```python
from build123d import *

# Parameters (mm, degrees)
F0_R     = 4.075
F1_DEPTH = 5
F2_R     = 8
F3_R     = 30
F4_W     = 8
F4_H     = 8
F5_DEPTH = 4
F6_R     = 1
F8_COUNT = 3
F8_ANGLE = 180
F9_SIZE  = 0.25


with BuildPart() as f1:
    # F0 (on Top) → F1 (new body)
    with BuildSketch(Plane.XY):
        Polygon((-14.5, 14.5), (-68, 14.5), (-68, -14.5), (0, -14.5), (68, -14.5), (68, 14.5), (14.5, 14.5), (14.5, 68), (-14.5, 68), align=None)
        with Locations((-60, 0)):
            Circle(F0_R, mode=Mode.SUBTRACT)
        with Locations((-30, 0)):
            Circle(F0_R, mode=Mode.SUBTRACT)
        Circle(F0_R, mode=Mode.SUBTRACT)
        with Locations((30, 0)):
            Circle(F0_R, mode=Mode.SUBTRACT)
        with Locations((60, 0)):
            Circle(F0_R, mode=Mode.SUBTRACT)
        with Locations((0, 30)):
            Circle(F0_R, mode=Mode.SUBTRACT)
        with Locations((0, 60)):
            Circle(F0_R, mode=Mode.SUBTRACT)
    extrude(amount=F1_DEPTH)

    # F2
    f2_edges = [f1.edges().sort_by_distance(p)[0] for p in [
        (-14.5, 68, 2.5),
        (14.5, 68, 2.5),
        (-68, 14.5, 2.5),
        (-68, -14.5, 2.5),
        (68, 14.5, 2.5),
        (68, -14.5, 2.5),
    ]]
    fillet(f2_edges, radius=F2_R)

    # F3
    f3_edges = [f1.edges().sort_by_distance(p)[0] for p in [
        (14.5, 14.5, 2.5),
        (-14.5, 14.5, 2.5),
    ]]
    fillet(f3_edges, radius=F3_R)



with BuildPart() as f5:
    # F4 (on face) → F5 (new body)
    with BuildSketch(Plane.XY.offset(5)):
        with Locations((-45, 0)):
            Rectangle(F4_W, F4_H)
    extrude(amount=F5_DEPTH)

    # F6
    f6_edges = [f5.edges().sort_by_distance(p)[0] for p in [
        (-49, -4, 7),
        (-41, -4, 7),
        (-49, 4, 7),
        (-41, 4, 7),
    ]]
    fillet(f6_edges, radius=F6_R)


with BuildPart() as f1_1:
    add(f1.part)

    add(f5.part)  # F8 merges F5
    # F8: F5 ×3 about axis
    f8_axis = Axis((0, 0, 11.3541549072), (0, 0, -1))
    for i in range(1, F8_COUNT):
        add(f5.part.rotate(f8_axis, i * F8_ANGLE / (F8_COUNT - 1)))

    # F9
    f9_edges = [f1_1.edges().sort_by_distance(p)[0] for p in [
        (-52.25, 14.5, 0),
        (-23.286797, 23.286797, 0),
        (-65.656854, 12.156854, 0),
        (-14.5, 52.25, 0),
        (-68, 0, 0),
        (-12.156854, 65.656854, 0),
        (-65.656854, -12.156854, 0),
        (0, 68, 0),
        (0, -14.5, 0),
        (12.156854, 65.656854, 0),
        (65.656854, -12.156854, 0),
        (14.5, 52.25, 0),
        (68, 0, 0),
        (23.286797, 23.286797, 0),
        (65.656854, 12.156854, 0),
        (52.25, 14.5, 0),
        (-64.075, 0, 0),
        (-34.075, 0, 0),
        (-4.075, 0, 0),
        (25.925, 0, 0),
        (55.925, 0, 0),
        (-4.075, 30, 0),
        (-4.075, 60, 0),
    ]]
    chamfer(f9_edges, length=F9_SIZE)


solid = f1_1.part
```
Here's how the part is built. I have some questions about the finished solid (model axes, mm). A direction names the side the tool comes from. Give positions to 0.01 mm unless a question says otherwise; leave off trailing zeros. Loops run counter-clockwise (first coordinate to the right, second up) from the corner with the lowest first, then second, coordinate; pieces in that order, holes last. Notation, with made-up numbers: M 48.25,18.5 L 65.25,18.5 A22 cw 65.25,46.5 Z; hole C -6,-37 d11. An arc over 180 degrees is marked long. Return JSON: item names as keys, results as strings.
Item 1: Thinking about a two-plate mould opening in X: for faces 5 (the flat face through (45, 0, 9)), 6 (the flat face through (14.5, 52, 3)), 7 (the cylindrical face through (63.89, 1.22, 2.59)), which applies, released by +X, released by -X, zero draft, split by the parting line, or undercut?
A:
{"face 5": "zero draft", "face 6": "released by +X", "face 7": "undercut"}
Item 2: On a 3-axis mill with a long thin cutter (end or side, diameter ignored), from which of +Z, -Z, +X, -X, +Y, -Y can I reach the whole of each face in a straight line? I mean faces 1 (the cylindrical face through (-3.003, 32.754, 2.592)), 2 (the flat face through (0, 49, 7)), 3 (the flat face through (-45, -4, 7)), 4 (the flat face through (-14.5, 52, 3)). Say none if no direction works.
A:
{"face 1": "+Z, -Z", "face 2": "+Z, +X, -X, +Y", "face 3": "+Z, +X, -X, -Y", "face 4": "+Z, -Z, -X, +Y"}
Item 3: Please list where these lines run through material, in increasing order: line 1 (Y direction, x = 0, z = 1.6) (3 decimals); line 2 (X direction, y = 47, z = 4.5); line 3 (Z direction, x = -4, y = 36.5).
A:
{"line 1": "y = -14.5 to -4.075, 4.075 to 25.925, 34.075 to 55.925, 64.075 to 68", "line 2": "x = -14.5 to 14.5", "line 3": "z = 0 to 5"}
Item 4: I'm going to push flat-ended pins straight in: pin 1 Ø2 at (y, z) = (0, 7.5) entering from +X; pin 2 Ø5 at (y, z) = (32, 6.5) entering from -X; pin 3 Ø1.4 at (x, z) = (-49, 2.5) entering from +Y. Where does each tip first touch, or does it pass through?
A:
{"pin 1": "stops at x = 49", "pin 2": "stops at x = -18.24", "pin 3": "stops at y = 14.5"}
Item 5: Imagine slicing it at C-C on y = 0. State how many separate pieces and enclosed holes the cut face has, then the cut area to 3 significant figures.
A:
{"separate pieces": "6", "enclosed holes": "0", "area": "540 mm^2"}
Item 6: Imagine slicing it at A-A on z = 6.5. List the corners of the cut face in (x, y) for me.
A:
{"outline": "M -49,-3 A1 ccw -48,-4 L -42,-4 A1 ccw -41,-3 L -41,3 A1 ccw -42,4 L -48,4 A1 ccw -49,3 Z; M -4,42 A1 ccw -3,41 L 3,41 A1 ccw 4,42 L 4,48 A1 ccw 3,49 L -3,49 A1 ccw -4,48 Z; M 41,-3 A1 ccw 42,-4 L 48,-4 A1 ccw 49,-3 L 49,3 A1 ccw 48,4 L 42,4 A1 ccw 41,3 Z"}
Item 7: Imagine slicing it at B-B on y = 52.5. List the corners of the cut face in (x, z) for me, then the cut area to 3 significant figures.
A:
{"outline": "M -14.5,0.25 L -14.25,0 L 14.25,0 L 14.5,0.25 L 14.5,5 L -14.5,5 Z", "area": "145 mm^2"}
